Geometry check sheet. Reference: the model listing, model coordinates, mm. A direction names the side the tool comes from. Round coordinates to 2 decimals unless told otherwise and drop trailing zeros. Order: outer loops, then holes, each group sorted by start corner. A loop starts at its lowest first (then second) coordinate and runs counter-clockwise, first axis right, second up. Notation, with made-up numbers: M 53.25,41.5 L 79.25,41.5 A30 cw 79.25,76.5 Z; hole C 17.25,8 d6. An arc over 180 degrees is marked long. Return JSON: item names as keys, results as strings. Group by question number.
```python
from build123d import *

# Parameters (mm, degrees)
SKETCH_1_W                       = 55
SKETCH_1_H                       = 60
EXTRUDE_1_DEPTH                  = 16.5
HOLE_WIZARD_3_6_3_6_1_D          = 3.6
HOLE_WIZARD_3_6_3_6_1_DEPTH      = 25
HOLE_WIZARD_3_6_3_6_1_TIP        = 1.081549114
HOLE_WIZARD_M2_5_1_D             = 2.05
HOLE_WIZARD_M2_5_1_DEPTH         = 14
HOLE_WIZARD_M2_5_1_TIP           = 0.615882135
SKETCH_8_W                       = 35
SKETCH_8_H                       = 20.4
CUT_EXTRUDE_1_DEPTH              = 44.914690025
CUT_EXTRUDE_START                = 2.5
SKETCH_9_W                       = 20
SKETCH_9_H                       = 6
CUT_EXTRUDE_2_DEPTH              = 42.414690025
SHELL_START                      = 1.8
SHELL_1_DEPTH                    = 14.7
EXTRUDE_2_DEPTH                  = 8
SKETCH_16_R                      = 3
CUT_EXTRUDE_4_DEPTH              = 12
CUT_EXTRUDE_5_DEPTH              = 47.599785407
CUT_EXTRUDE_5_DEPTH_BACK         = 47.599785407
SKETCH_17_R                      = 10
FILLET_1_R                       = 0.5
FILLET_2_R                       = 0.5
SKETCH_20_W                      = 1.8
SKETCH_20_H                      = 8
HOLE_WIZARD_3_6_3_6_2_AT_2_COUNT = 2
HOLE_WIZARD_3_6_3_6_2_AT_2_PITCH = 27.5
HOLE_WIZARD_3_6_3_6_2_AT_3_COUNT = 2
HOLE_WIZARD_3_6_3_6_2_AT_3_PITCH = 61.846584384
HOLE_WIZARD_3_6_3_6_2_AT_4_COUNT = 2
HOLE_WIZARD_3_6_3_6_2_AT_4_PITCH = 48
CUT_EXTRUDE_6_DEPTH              = 2
FILLET_3_R                       = 2
EXTRUDE_START                    = -8
SKETCH_24_R                      = 15
SKETCH_24_R_2                    = 10
EXTRUDE_3_DEPTH                  = 20
CHAMFER_1_SIZE                   = 0.5
CUT_EXTRUDE_START_2              = -2
SKETCH_25_R                      = 12.3
CUT_EXTRUDE_7_DEPTH              = 3
SKETCH_26_R                      = 12
CUT_EXTRUDE_8_DEPTH              = 12
SKETCH_27_W                      = 27.90091823
SKETCH_27_H                      = 2.950248151
CUT_EXTRUDE_9_DEPTH              = 12


# Read off the part's stored shape, not the designer's step: 抽壳1
with BuildPart() as part:
    # 草图1 → 凸台-拉伸1 (new body)
    with BuildSketch(Plane.XY):
        Rectangle(SKETCH_1_W, SKETCH_1_H)
    extrude(amount=EXTRUDE_1_DEPTH)

    # Ø3.6 (3.6) 直径孔1
    with Locations(Plane.XY.offset(16.5)):
        with Locations((-24, 21.5), (24, 21.5), (24, -6), (-15, -26.5)):
            Hole(HOLE_WIZARD_3_6_3_6_1_D / 2, depth=HOLE_WIZARD_3_6_3_6_1_DEPTH)
            with Locations((0, 0, -(HOLE_WIZARD_3_6_3_6_1_DEPTH + HOLE_WIZARD_3_6_3_6_1_TIP / 2))):  # 118° drill point
                Cone(0, HOLE_WIZARD_3_6_3_6_1_D / 2, HOLE_WIZARD_3_6_3_6_1_TIP, mode=Mode.SUBTRACT)

    # M2.5 螺纹孔1
    with Locations(Plane.XY.offset(16.5)):
        with Locations((-24, 26.5), (24, 26.5), (24, -1), (-22.5, -26.5)):
            Hole(HOLE_WIZARD_M2_5_1_D / 2, depth=HOLE_WIZARD_M2_5_1_DEPTH)
            with Locations((0, 0, -(HOLE_WIZARD_M2_5_1_DEPTH + HOLE_WIZARD_M2_5_1_TIP / 2))):  # 118° drill point
                Cone(0, HOLE_WIZARD_M2_5_1_D / 2, HOLE_WIZARD_M2_5_1_TIP, mode=Mode.SUBTRACT)

    # 草图8 → 切除-拉伸1 (cut, through all)
    with BuildSketch(Plane.XY.offset(16.5)):
        with Locations((10, -19.8)):
            Rectangle(SKETCH_8_W, SKETCH_8_H)
    extrude(amount=-CUT_EXTRUDE_1_DEPTH, mode=Mode.SUBTRACT)

    # 草图9 → 切除-拉伸2 (cut, through all)
    with BuildSketch(Plane(origin=(0, 0, 16.5), x_dir=(-1, 0, 0), z_dir=(0, 0, -1)).offset(CUT_EXTRUDE_START)):
        with Locations((17.5, -27)):
            Rectangle(SKETCH_9_W, SKETCH_9_H)
    extrude(amount=CUT_EXTRUDE_2_DEPTH, mode=Mode.SUBTRACT)

    # 抽壳1 outline → 抽壳1 (cut)
    with BuildSketch(Plane.XY.offset(SHELL_START)):
        with BuildLine():
            ThreePointArc((-21.743758657, 28.2), (-21.182110509, 26.299690696), (-22.006919283, 24.4979375))
            ThreePointArc((-22.006919283, 24.4979375), (-20.910890356, 19.651378458), (-25.7, 18.326673669))
            Line((-25.7, 18.326673669), (-25.7, -22.2))
            Line((-25.7, -22.2), (-9.3, -22.2))
            Line((-9.3, -22.2), (-9.3, -7.8))
            Line((-9.3, -7.8), (20.882308546, -7.8))
            ThreePointArc((20.882308546, -7.8), (20.494996561, -5.178446051), (22.006919283, -3.0020625))
            ThreePointArc((22.006919283, -3.0020625), (21.865811165, 0.8509087), (25.7, 1.256241343))
            Line((25.7, 1.256241343), (25.7, 18.326673669))
            ThreePointArc((25.7, 18.326673669), (20.910890356, 19.651378458), (22.006919283, 24.4979375))
            ThreePointArc((22.006919283, 24.4979375), (21.182110509, 26.299690696), (21.743758657, 28.2))
            Line((21.743758657, 28.2), (-21.743758657, 28.2))
        make_face()
    extrude(amount=SHELL_1_DEPTH, mode=Mode.SUBTRACT)

    # 草图16 → 切除-拉伸4 (cut)
    with BuildSketch(Plane(origin=(-7.5, 0, 0), x_dir=(0, 0, -1), z_dir=(1, 0, 0))):
        with Locations(Location((-8, -18, 0), (0, 0, 90))):
            Circle(SKETCH_16_R)
    extrude(amount=-CUT_EXTRUDE_4_DEPTH, mode=Mode.SUBTRACT)


with BuildPart() as body_2:
    # 草图10 → 凸台-拉伸2 (new body)
    with BuildSketch(Plane.XY.offset(16.5)):
        Polygon((-27.5, -30), (-7.5, -30), (-7.5, -9.6), (27.5, -9.6), (27.5, 30), (-27.5, 30), align=None)
    extrude(amount=EXTRUDE_2_DEPTH)


with BuildPart() as cut_extrude_5_tool:
    # 草图17 → 切除-拉伸5 (new, two sides: drawn at the far end of the back side and taken through both)
    with BuildSketch(Plane.XY.offset(1.8).offset(-CUT_EXTRUDE_5_DEPTH_BACK)):
        with Locations((6.5, 9.5)):
            Circle(SKETCH_17_R)
    extrude(amount=CUT_EXTRUDE_5_DEPTH + CUT_EXTRUDE_5_DEPTH_BACK)


with BuildPart() as part_1:
    add(part.part)

    # 切除-拉伸5: cut by cut_extrude_5_tool
    add(cut_extrude_5_tool.part, mode=Mode.SUBTRACT)

    # 圆角1
    fillet_1_edges = [part_1.edges().sort_by_distance(p)[0] for p in [
        (-27.5, 3, 0),
        (0, 30, 0),
        (27.5, 10.2, 0),
        (27.5, -9.6, 8.25),
        (-7.5, -16.8, 0),
        (10, -9.6, 0),
        (-7.5, -9.6, 8.25),
        (-7.5, -30, 15.25),
        (-27.5, -30, 15.25),
        (-27.5, 30, 8.25),
        (27.5, 30, 8.25),
        (-17.5, -24, 0),
        (-7.5, -24, 7),
        (-27.5, -24, 7),
    ]]
    fillet(fillet_1_edges, radius=FILLET_1_R)


with BuildPart() as body_2_1:
    add(body_2.part)

    # 切除-拉伸5: cut by cut_extrude_5_tool
    add(cut_extrude_5_tool.part, mode=Mode.SUBTRACT)

    # 圆角2
    fillet_2_edges = [body_2_1.edges().sort_by_distance(p)[0] for p in [
        (-27.5, 30, 20.5),
        (27.5, 30, 20.5),
        (27.5, -9.6, 20.5),
        (-7.5, -9.6, 20.5),
        (-7.5, -30, 20.5),
        (-27.5, -30, 20.5),
    ]]
    fillet(fillet_2_edges, radius=FILLET_2_R)

    # 草图20 → Ø3.6 (3.6) 直径孔2 (revolve, cut)
    with BuildSketch(Plane(origin=(24, 21.5, 16.5), x_dir=(0, 1, 0), z_dir=(1, 0, 0))):
        with Locations((0.9, 4)):
            Rectangle(SKETCH_20_W, SKETCH_20_H)
    hole_wizard_3_6_3_6_2 = revolve(axis=Axis((24, 21.5, 10.15), (0, 0, 1)), mode=Mode.SUBTRACT)

    # Ø3.6 (3.6) 直径孔2 at 2: Ø3.6 (3.6) 直径孔2 ×2
    with Locations(*[(0, -i * HOLE_WIZARD_3_6_3_6_2_AT_2_PITCH, 0) for i in range(1, HOLE_WIZARD_3_6_3_6_2_AT_2_COUNT)]):
        add(hole_wizard_3_6_3_6_2, mode=Mode.SUBTRACT)

    # Ø3.6 (3.6) 直径孔2 at 3: Ø3.6 (3.6) 直径孔2 ×2
    with Locations(*[Vector(-0.6305926250944656, -0.7761140001162656, 0) * (i * HOLE_WIZARD_3_6_3_6_2_AT_3_PITCH) for i in range(1, HOLE_WIZARD_3_6_3_6_2_AT_3_COUNT)]):
        add(hole_wizard_3_6_3_6_2, mode=Mode.SUBTRACT)

    # Ø3.6 (3.6) 直径孔2 at 4: Ø3.6 (3.6) 直径孔2 ×2
    with Locations(*[(-i * HOLE_WIZARD_3_6_3_6_2_AT_4_PITCH, 0, 0) for i in range(1, HOLE_WIZARD_3_6_3_6_2_AT_4_COUNT)]):
        add(hole_wizard_3_6_3_6_2, mode=Mode.SUBTRACT)

    # 草图23 → 切除-拉伸6 (cut)
    with BuildSketch(Plane(origin=(0, 0, 16.5), x_dir=(-1, 0, 0), z_dir=(0, 0, -1))):
        with BuildLine():
            Line((8.25, -10.1), (8.25, -29.25))
            Line((8.25, -29.25), (26.75, -29.25))
            Line((26.75, -29.25), (26.75, 29.25))
            Line((26.75, 29.25), (-26.75, 29.25))
            Line((-26.75, 29.25), (-26.75, -8.85))
            Line((-26.75, -8.85), (7, -8.85))
            ThreePointArc((7, -8.85), (7.883883476, -9.216116524), (8.25, -10.1))
        make_face()
    extrude(amount=-CUT_EXTRUDE_6_DEPTH, mode=Mode.SUBTRACT)

    # 圆角3
    fillet_3_edges = [body_2_1.edges().sort_by_distance(p)[0] for p in [
        (26.75, -8.85, 17.5),
        (26.75, 29.25, 17.5),
        (-26.75, 29.25, 17.5),
        (-26.75, -29.25, 17.5),
        (-8.25, -29.25, 17.5),
    ]]
    fillet(fillet_3_edges, radius=FILLET_3_R)

    # 草图24 → 凸台-拉伸3 (add)
    with BuildSketch(Plane(origin=(0, 0, 18.5), x_dir=(-1, 0, 0), z_dir=(0, 0, -1)).offset(EXTRUDE_START)):
        with Locations((-6.5, 9.5)):
            Circle(SKETCH_24_R)
        with Locations((-6.5, 9.5)):
            Circle(SKETCH_24_R_2, mode=Mode.SUBTRACT)
    extrude(amount=EXTRUDE_3_DEPTH)

    # 倒角1
    chamfer_1_edges = [body_2_1.edges().sort_by_distance(p)[0] for p in [
        (21.5, 9.5, 26.5),
        (21.5, 9.5, 6.5),
        (16.5, 9.5, 26.5),
    ]]
    chamfer(chamfer_1_edges, length=CHAMFER_1_SIZE)

    # 草图25 → 切除-拉伸7 (cut)
    with BuildSketch(Plane.XY.offset(26.5).offset(CUT_EXTRUDE_START_2)):
        with Locations((6.5, 9.5)):
            Circle(SKETCH_25_R)
    extrude(amount=-CUT_EXTRUDE_7_DEPTH, mode=Mode.SUBTRACT)

    # 草图26 → 切除-拉伸8 (cut)
    with BuildSketch(Plane(origin=(0, 0, 6.5), x_dir=(-1, 0, 0), z_dir=(0, 0, -1))):
        with Locations((-6.5, 9.5)):
            Circle(SKETCH_26_R)
    extrude(amount=-CUT_EXTRUDE_8_DEPTH, mode=Mode.SUBTRACT)

    # 草图27 → 切除-拉伸9 (cut)
    with BuildSketch(Plane(origin=(0, 0, 6.5), x_dir=(-1, 0, 0), z_dir=(0, 0, -1))):
        with Locations((-4.79900427, -5.825124076)):
            Rectangle(SKETCH_27_W, SKETCH_27_H)
        with Locations((-4.79900427, 24.825124075)):
            Rectangle(SKETCH_27_W, SKETCH_27_H)
    extrude(amount=-CUT_EXTRUDE_9_DEPTH, mode=Mode.SUBTRACT)


solid = body_2_1.part
```
Q1. Material ranges on line 1 along X through (y, z) = (-6, 22.1); line 2 along Y through (x, z) = (6.5, 25.2); line 3 along Z through (x, y) = (2, -1.5), recorded low to high.
Q2. Section check B-B on x = 24. Record the cut outline in (y, z).
Q3. Section check A-A on z = 17.5. Count the separate pieces of the cut face and the enclosed holes in it, plus the area to 3 significant figures.
Q4. Set-up check for faces 4 (the face through (26.75, 10, 17)), 5 (the face through (-27.5, 0, 20)): record each of +Z, -Z, +X, -X, +Y, -Y from which the full face is reachable in a straight line by a thin tool's end or side.
Q5. Depth check by flat-ended pin: pin 1 Ø3 at (y, z) = (-17, 17.5) entering from +X; pin 2 Ø3 at (y, z) = (14.5, 10.5) entering from -X; pin 3 Ø0.6 at (x, z) = (11.5, 17) entering from -Y; pin 4 Ø3 at (x, y) = (24, -6) entering from +Z. Enter the tip coordinate at first touch or a pass-through.
Q6. Release check for a two-part mould opening along Z. For faces 1 (the face through (26.15, -8.28, 17.51)), 2 (the face through (21.133, 9.76, 6.635)), 3 (the face through (6, 20, 21.5)) record: +Z half, -Z half, draft (parallel to the pull), parting line (faces both ways), or undercut.
Q7. Section check D-D on y = -14. Record the cut outline in (x, z).
Q8. Section check C-C on x = -15. Record the cut outline in (y, z).
Geometry check:
{
 "1": {"line 1": "x = -27.5 to 22.2, 25.8 to 27.5", "line 2": "y = -5.5 to -0.5, 19.5 to 24.5", "line 3": "z = 18.5 to 21.5, 24.5 to 26.5"},
 "2": {"outline": "M -9.6,16.5 L -8.85,16.5 L -8.85,18.5 L -7.8,18.5 L -7.8,24.5 L -9.6,24.5 Z; M -4.2,18.5 L 19.7,18.5 L 19.7,24.5 L -4.2,24.5 Z; M 23.3,18.5 L 29.25,18.5 L 29.25,16.5 L 30,16.5 L 30,24.5 L 23.3,24.5 Z"},
 "3": {"separate pieces": "2", "enclosed holes": "2", "area": "411 mm^2"},
 "4": {"face 4": "-Z", "face 5": "+Z, -Z, -X, +Y, -Y"},
 "5": {"pin 1": "stops at x = -7.5", "pin 2": "stops at x = -8.09", "pin 3": "stops at y = -9.6", "pin 4": "passes through"},
 "6": {"face 1": "draft", "face 2": "-Z half", "face 3": "undercut"},
 "7": {"outline": "M -27.5,16.5 L -26.75,16.5 L -26.75,18.5 L -8.25,18.5 L -8.25,16.5 L -7.5,16.5 L -7.5,24.5 L -27.5,24.5 Z"},
 "8": {"outline": "M -30,16.5 L -29.25,16.5 L -29.25,18.5 L -28.3,18.5 L -28.3,24.5 L -30,24.5 Z; M -24.7,18.5 L 29.25,18.5 L 29.25,16.5 L 30,16.5 L 30,24.5 L -24.7,24.5 Z"}
}
